Geometry: see drawing. Coordinates: mm, zero at the bounding-box minimum. A direction names the side the tool comes from. Coordinates: 2 decimals unless noted, no trailing zeros. Order: outer loops, then holes, each group sorted by start corner. A loop starts at its lowest first (then second) coordinate and runs counter-clockwise, first axis right, second up.
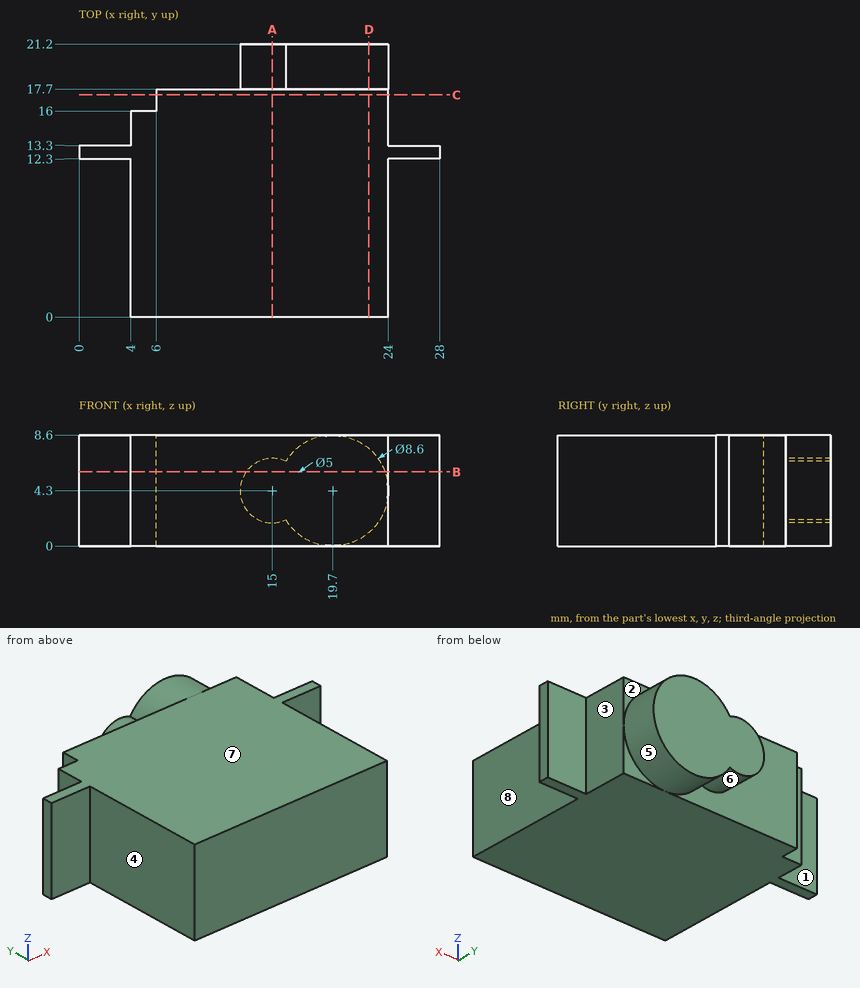
Q1. Section query B-B on z = 5.75. Output: boundary loops of the cut face in (x, y).
Solutions:
outline: (0, 12.3) - (4, 12.3) - (4, 0) - (24, 0) - (24, 12.3) - (28, 12.3) - (28, 13.3) - (24, 13.3) - (24, 17.7) - (23.75, 17.7) - (23.75, 21.2) - (12.96, 21.2) - (12.96, 17.7) - (6, 17.7) - (6, 16) - (4, 16) - (4, 13.3) - (0, 13.3) - close
Q2. Pull-direction query (X, two-part tool) for the marked faces 6, 7 and 8; classes: pulls with the +X half, pulls with the -X half, needs draft (parallel to the pull), parting line crosses it, or undercut.
Solutions:
face 6: undercut
face 7: needs draft
face 8: pulls with the +X half
Q3. Section query D-D on x = 22.5. Output: boundary loops of the cut face in (y, z).
Solutions:
outline: (0, 0) - (17.7, 0) - (17.7, 1.04) - (21.2, 1.04) - (21.2, 7.56) - (17.7, 7.56) - (17.7, 8.6) - (0, 8.6) - close
Q4. Section query C-C on y = 17.25. Output: boundary loops of the cut face in (x, z), plus the area to 3 significant figures.
Solutions:
outline: (6, 0) - (24, 0) - (24, 8.6) - (6, 8.6) - close
area: 155 mm2
Q5. Material intervals for line 1 along Y through (x, z) = (22.75, 7.5); line 2 along X through (y, z) = (12, 1); line 3 along X through (y, z) = (16.75, 1.5), sorted ascending.
Solutions:
line 1: y = 0 to 17.7
line 2: x = 4 to 24
line 3: x = 6 to 24
Q6. Section query A-A on x = 15. Output: boundary loops of the cut face in (y, z).
Solutions:
outline: (0, 0) - (17.7, 0) - (17.7, 1.8) - (21.2, 1.8) - (21.2, 6.8) - (17.7, 6.8) - (17.7, 8.6) - (0, 8.6) - close
Q7. Set-up query: the marked faces 1, 2, 3, 4 and 5. Return all of +Z, -Z, +X, -X, +Y, -Y with unobstructed straight access to the full face (end or side cutting, diameter ignored); none if empty.
Solutions:
face 1: +Z, -Z, -X, +Y
face 2: +Z, +X, +Y
face 3: +Z, -Z, +X, +Y
face 4: +Z, -Z, -X, -Y
face 5: +Y
Q8. Pin query (flat end, axial travel): P1, Ø0.6, axis at x = 5, z = 4, coming from the +Y side; P2, Ø2, axis at x = 2.5, z = 4.5, coming from the +Y side; P3, Ø1.3, axis at y = 16, z = 2.5, coming from the +X side. Return the tip coordinate at first contact, or that it passes through.
Solutions:
P1: stops at y = 16
P2: stops at y = 13.3
P3: stops at x = 24
